```python
from build123d import *

# Parameters (mm, degrees)
F0_W     = 76.2
F0_H     = 76.2
F1_DEPTH = 25.4
F2_W     = 50.8
F2_H     = 50.8
F2_R     = 3.175
F3_DEPTH = 19.05
F4_R     = 5.08
F5_R     = 3.175
F6_DEPTH = 12.7
F7_DEPTH = 6.35


with BuildPart() as f1:
    # F0 (on Top) → F1 (new body)
    with BuildSketch(Plane.XY):
        with Locations((-0.2496400848, -1.4978470281)):
            Rectangle(F0_W, F0_H)
    extrude(amount=F1_DEPTH)

    # F2 (on face) → F3 (cut)
    with BuildSketch(Plane.XY.offset(25.4)):
        with Locations((-0.2496400848, -1.4978470281)):
            Rectangle(F2_W, F2_H)
        with Locations((-31.9996400848, -33.2478470281)):
            Circle(F2_R)
        with Locations((31.5003599152, -33.2478470281)):
            Circle(F2_R)
        with Locations((31.5003599152, 30.2521529719)):
            Circle(F2_R)
        with Locations((-31.9996400848, 30.2521529719)):
            Circle(F2_R)
    extrude(amount=-F3_DEPTH, mode=Mode.SUBTRACT)

    # F4
    f4_edges = [f1.edges().sort_by_distance(p)[0] for p in [
        (-38.34964, 36.602153, 12.7),
        (37.85036, 36.602153, 12.7),
        (37.85036, -39.597847, 12.7),
        (-38.34964, -39.597847, 12.7),
        (25.15036, 23.902153, 15.875),
        (25.15036, -26.897847, 15.875),
        (-25.64964, -26.897847, 15.875),
        (-25.64964, 23.902153, 15.875),
    ]]
    fillet(f4_edges, radius=F4_R)

    # F5 (on face) → F6 (cut, through all)
    with BuildSketch(Plane(origin=(25.1503599152, 0, 0), x_dir=(0, -1, 0), z_dir=(-1, 0, 0))):
        with Locations((0, 15.875)):
            Circle(F5_R)
    extrude(amount=-F6_DEPTH, mode=Mode.SUBTRACT)

    # F7 (cut, through all): faces of the model
    f7_faces = [f1.faces().sort_by_distance(p)[0] for p in [
        (31.5003599152, 30.2521529719, 6.35),
        (31.5003599152, -33.2478470281, 6.35),
        (-31.9996400848, 30.2521529719, 6.35),
        (-31.9996400848, -33.2478470281, 6.35),
    ]]
    extrude(f7_faces, amount=-F7_DEPTH, mode=Mode.SUBTRACT)


solid = f1.part
```
Here's how the part is built. I have some questions about the finished solid (model axes, mm). A direction names the side the tool comes from. Coordinates: 2 decimals unless noted, no trailing zeros. Write each loop counter-clockwise with the first axis right and the second up, starting at its lowest first coordinate (ties: lowest second). Pieces come first, ordered by that corner, then holes. Notation, with made-up numbers: (31, 68) - (64, 68) arc R21 ccw to (64, 78) - close; hole circle Ø2 at (78, -36). An arc over 180 degrees is marked (long way). One line per item, written item: value.
1) We'd pull the mould along X, two halves only. Please class faces 1 (the flat face through (37.85, -2, 13)), 2 (the flat face through (-38.35, -2, 13)), 3 (the cylindrical face through (31.1, 33.4, 12.9)): pulls with the +X half, pulls with the -X half, needs draft (parallel to the pull), parting line crosses it, or undercut.
Model answer:
face 1: pulls with the +X half
face 2: pulls with the -X half
face 3: undercut
2) Suppose I cut it at D-D on y = -10.5. Write out the boundary of the cut face in (x, z).
Model answer:
outline: (-38.35, 0) - (37.85, 0) - (37.85, 25.4) - (25.15, 25.4) - (25.15, 6.35) - (-25.65, 6.35) - (-25.65, 25.4) - (-38.35, 25.4) - close
3) Suppose I cut it at B-B on y = 0. Write out the boundary of the cut face in (x, z).
Model answer:
outline: (-38.35, 0) - (37.85, 0) - (37.85, 12.7) - (25.15, 12.7) - (25.15, 6.35) - (-25.65, 6.35) - (-25.65, 25.4) - (-38.35, 25.4) - close; (25.15, 19.05) - (37.85, 19.05) - (37.85, 25.4) - (25.15, 25.4) - close
4) I'm going to push flat-ended pins straight in: P1, Ø1, axis at x = 9.5, y = -6.5, coming from the -Z side; P2, Ø8, axis at x = -0.5, y = 0.5, coming from the +Z side; P3, Ø5.5, axis at x = 31.5, y = -33.25, coming from the +Z side. Where does each tip first touch, or does it pass through?
Model answer:
P1: stops at z = 0
P2: stops at z = 6.35
P3: passes through
5) On a 3-axis mill with a long thin cutter (end or side, diameter ignored), from which of +Z, -Z, +X, -X, +Y, -Y can I reach the whole of each face in a straight line? I mean faces 4 (the cylindrical face through (31.411, 0.413, 19.023)), 5 (the cylindrical face through (-24.12, -25.45, 15.74)), 6 (the flat face through (-1, -39.598, 13)). Say none if no direction works.
Model answer:
face 4: +X
face 5: +Z
face 6: +Z, -Z, +X, -X, -Y
6) I need wall thicknesses on line 1 along X through (y, z) = (-33, 9.25); line 2 along X through (y, z) = (16.5, 11.5); line 3 along Y through (x, z) = (6.5, 11.5). Which ranges of each line are inside material? Lowest first, please.
Model answer:
line 1: x = -38.35 to -35.16, -28.83 to 28.34, 34.67 to 37.85
line 2: x = -38.35 to -25.65, 25.15 to 37.85
line 3: y = -39.6 to -26.9, 23.9 to 36.6
7) Suppose I cut it at A-A on x = -32. Write out the boundary of the cut face in (y, z).
Model answer:
outline: (-39.6, 0) - (-36.42, 0) - (-36.42, 25.4) - (-39.6, 25.4) - close; (-30.07, 0) - (27.08, 0) - (27.08, 25.4) - (-30.07, 25.4) - close; (33.43, 0) - (36.6, 0) - (36.6, 25.4) - (33.43, 25.4) - close
8) Suppose I cut it at C-C on z = 21.75. Write out the boundary of the cut face in (x, y) (3 decimals).
Model answer:
outline: (-38.35, -34.518) arc R5.08 ccw to (-33.27, -39.598) - (32.77, -39.598) arc R5.08 ccw to (37.85, -34.518) - (37.85, 31.522) arc R5.08 ccw to (32.77, 36.602) - (-33.27, 36.602) arc R5.08 ccw to (-38.35, 31.522) - close; hole circle Ø6.35 at (-32, -33.248); hole circle Ø6.35 at (-32, 30.252); hole (-25.65, -21.818) arc R5.08 ccw to (-20.57, -26.898) - (20.07, -26.898) arc R5.08 ccw to (25.15, -21.818) - (25.15, 18.822) arc R5.08 ccw to (20.07, 23.902) - (-20.57, 23.902) arc R5.08 ccw to (-25.65, 18.822) - close; hole circle Ø6.35 at (31.5, -33.248); hole circle Ø6.35 at (31.5, 30.252)
